Input: part model. Units: mm. Frame: model coordinates. A direction names the side the tool comes from. Round coordinates to 2 decimals unless told otherwise and drop trailing zeros. Order: outer loops, then holes, each group sorted by start corner. A loop starts at its lowest first (then second) coordinate and runs counter-clockwise, first axis right, second up. Notation, with made-up numbers: M 9,20.25 L 53,20.25 A20 cw 53,36.25 Z; hole C 58,81 d11. An arc over 180 degrees is marked long. One line per question, with ' | ' between items.
Autodesk Inventor part; units mm, degrees
ref_plane "YZ Plane" through (0, 0, 0) normal (1, 0, 0) x (0, 1, 0)
ref_plane "XZ Plane" through (0, 0, 0) normal (0, 1, 0) x (-1, 0, 0)
ref_plane "XY Plane" through (0, 0, 0) normal (0, 0, 1) x (1, 0, 0)
sketch "Sketch1" plane through (0, 0, 0) normal (0, 1, 0) x (-1, 0, 0)
  line L0 (17.0295, 14.999) -> (-8.3705, 14.999)
  line L1 (-8.3705, 14.999) -> (-8.3705, -10.401)
  line L2 (-8.3705, -10.401) -> (17.0295, -10.401)
  line L3 (17.0295, -10.401) -> (17.0295, 14.999)
  line L4 (15.442, -8.8135) -> (-6.783, -8.8135)
  line L5 (-6.783, -8.8135) -> (-6.783, 13.4115)
  line L6 (-6.783, 13.4115) -> (15.442, 13.4115)
  line L7 (15.442, 13.4115) -> (15.442, -8.8135)
  point P0 (0, 0)
  dimension "d0" = 25.4
  dimension "d1" = 25.4
  dimension "d4" = 1.5875
  dimension "d5" = 1.5875
  dimension "d6" = 1.5875
  dimension "d7" = 1.5875
extrude "Extrusion2" add sketch "Sketch1" along normal blind 990.6
sketch "Sketch4" plane through (8.3705, 0, 14.999) normal (1, 0, 0) x (0, 0, -1)
  line L0 (25.4, 0) -> (25.4, 990.6)
  line L1 (0, 990.6) -> (25.4, 990.6)
  point P0 (14.999, 0)
  point P1 (12.7, 939.8)
  dimension "d28" = 12.7
  dimension "d29" = 50.8
hole "Hole3" at (8.3705, 939.8, 2.299) direction (-1, 0, 0) diameter 9.5758 depth 25.4 tip angle 118
sketch "Sketch5" plane through (8.3705, 0, 14.999) normal (1, 0, 0) x (0, 0, -1)
  line L0 (0, 0) -> (0, 990.6)
  line L1 (0, 990.6) -> (25.4, 990.6)
  point P0 (14.999, 0)
  point P1 (12.7, 901.7)
  point P2 (12.7, 876.3)
  point P3 (12.7, 850.9)
  dimension "d37" = 25.4
  dimension "d38" = 25.4
  dimension "d39" = 12.7
  dimension "d40" = 12.7
  dimension "d41" = 12.7
  dimension "d42" = 88.9
hole "Hole4" at (8.3705, 901.7, 2.299) at (8.3705, 876.3, 2.299) at (8.3705, 850.9, 2.299) direction (-1, 0, 0) diameter 4.826 depth 25.4 tip angle 118
sketch "Sketch6" plane through (-17.0295, 0, 14.999) normal (0, 0, 1) x (1, 0, 0)
  line L0 (0, 0) -> (0, 990.6)
  line L1 (0, 990.6) -> (25.4, 990.6)
  line L2 (25.4, 0) -> (25.4, 990.6)
  point P0 (17.0295, 0)
  point P1 (6.35, 984.25)
  point P2 (19.05, 971.55)
  point P3 (6.35, 958.85)
  point P4 (19.05, 946.15)
  dimension "d50" = 6.35
  dimension "d51" = 6.35
  dimension "d52" = 6.35
  dimension "d53" = 25.4
  dimension "d54" = 6.35
  dimension "d55" = 19.05
  dimension "d56" = 6.35
  dimension "d57" = 25.4
hole "Hole5" at (-10.6795, 984.25, 14.999) at (2.0205, 971.55, 14.999) at (-10.6795, 958.85, 14.999) at (2.0205, 946.15, 14.999) direction (0, 0, -1) diameter 4.7625 depth 25.4 tip angle 118
sketch "Sketch7" plane through (-17.0295, 0, 14.999) normal (0, 0, 1) x (1, 0, 0)
  line L0 (25.4, 0) -> (25.4, 990.6)
  line L1 (0, 0) -> (25.4, 0)
  line L2 (0, 0) -> (0, 990.6)
  point P0 (17.0295, 0)
  point P1 (19.05, 31.75)
  point P2 (19.05, 57.15)
  point P3 (6.35, 44.45)
  point P4 (6.35, 69.85)
  dimension "d65" = 6.35
  dimension "d66" = 31.75
  dimension "d67" = 6.35
  dimension "d68" = 25.4
  dimension "d69" = 6.35
  dimension "d70" = 6.35
  dimension "d71" = 25.4
  dimension "d72" = 44.45
hole "Hole6" at (2.0205, 31.75, 14.999) at (2.0205, 57.15, 14.999) at (-10.6795, 44.45, 14.999) at (-10.6795, 69.85, 14.999) direction (0, 0, -1) diameter 4.7625 depth 25.4 tip angle 118
equation "\"d0\" = ElvBeamWidth"
equation "\"d1\" = ElvBeamWidth"
equation "\"d4\" = ElvWallWidth"
equation "\"d5\" = ElvWallWidth"
equation "\"d6\" = ElvWallWidth"
equation "\"d7\" = ElvWallWidth"
equation "\"d8\" = ElvFrontBeamLength"
equation "\"ElvMiddleBeamLength\" = 990.6"
equation "\"ElvWallWidth\" = 1.5875"
equation "\"ElvFrontBeamLength\" = 990.6"
equation "\"ElvEndEffectLength\" = 431.8"
equation "\"ElvCrossBeamLength\" = 304.8"
equation "\"ElvBeamWidth\" = 25.4"
equation "\"ElvFrontBeamLength_1\" = 1066.8"
equation "\"ElvFixedBeamLength\" = 990.6"
equation "\"ElvDelHeight\" = 101.6"
equation "\"ElvDelDepth\" = 6.35"
equation "\"ElvDelFrontTabLength\" = 6.35"
equation "\"ElvDelWidth\" = 18.542"
equation "\"ElvTopBeamLength\" = 457.2"
equation "\"ElvHoleFromBottom\" = 38.1"
equation "\"ElvHoleFromFront\" = 25.4"
equation "\"ElvHoleFromMid\" = 38.1"
equation "\"ElvHoleFromFixed\" = 50.8"
equation "\"ElvRivetPlateLength\" = 76.2"
equation "\"ElvDelMiddleTabLength\" = 6.35"
properties part number "ElvFixedBeam" material "Aluminum 6061"
Item 1: Mould query, pull axis X, two halves, no side actions, for faces 1 (the flat face through (8.37, 488, 2)), 2 (the flat face through (-17.03, 488, 2)), 3 (the flat face through (7, 0, 2)), 4 (the flat face through (-4, 488, 13.412)). Classes: +X half, -X half, draft (parallel to the pull), parting line (faces both ways), or undercut.
Report:
face 1: +X half | face 2: -X half | face 3: draft | face 4: undercut
Item 2: Section query A-A, the plane y = 360. Return loops of the section in (x, z).
Report:
outline: M -17.03,-10.4 L 8.37,-10.4 L 8.37,15 L -17.03,15 Z; hole M -15.44,-8.81 L 6.78,-8.81 L 6.78,13.41 L -15.44,13.41 Z
Item 3: Access query for faces 5 (the flat face through (6.783, 488, 2)), 6 (the flat face through (-4, 488, -10.401)). Directions: +Z, -Z, +X, -X, +Y, -Y. A direction counts if a zero-diameter tool reaches every point of the face in a straight line with its end or side. Return the directions, or none.
Report:
face 5: +Y, -Y | face 6: -Z, +X, -X, +Y, -Y
Item 4: Line query: line 1 along X through (y, z) = (971.55, 13.9); line 2 along Z through (x, y) = (6.5, 288.5); line 3 along X through (y, z) = (824.5, 13.25). Output: solid intervals per line, ascending. Write a range as from..to.
Report:
line 1: -17.03..-0.36, 4.4..8.37 | line 2: -10.4..-8.81, 13.41..15 | line 3: -17.03..-15.44, 6.78..8.37
Item 5: First-contact query: pin 1 (4.5 mm diameter, centred on x = -10.68, y = 69.85, fed in from +Z). Flat tip, straight axial feed; report the tip coordinate or a pass-through.
Report:
pin 1: through
